Check sheet for the drawn part. Datum: minimum x, y, z corner. Units: mm. Give positions to 0.01 mm unless a question says otherwise; leave off trailing zeros. Order: outer loops, then holes, each group sorted by start corner. A loop starts at its lowest first (then second) coordinate and runs counter-clockwise, first axis right, second up. Notation, with made-up numbers: (37.25, -3.5) -> (82.25, -3.5) arc R10 cw to (82.25, 2.5) -> close; hole circle Ø2 at (57, 80.25). An arc over 180 degrees is marked (long way). Answer in a Markdown table with one row per item. Add a question column.
(1) Go/stop test with flat-tipped pins: pin 1 (5 mm diameter, centred on x = 25, z = 4.76, fed in from -Y); pin 2 (3.5 mm diameter, centred on x = 25, z = 29.3, fed in from +Y). Record where each tip stops, or that it passes through.
(2) Cross-section at B-B (z = 29.3). Record the cut outline in (x, y) (1 decimal), then the cut area to 3 significant figures.
(3) Thickness scan on L1, parallel to X at y = 5.5, z = 29; L2, parallel to Z at x = 42, y = 4.5 (1 decimal); L3, parallel to Z at x = 41.67, y = 6.5. Record the ranges inside material, lowest first. Write a range as [from, to].
(4) Cross-section at C-C (y = 7.75). State how many separate pieces and enclosed holes the cut face has, then the cut area to 3 significant figures.
(5) Cross-section at A-A (x = 41.67). Record the cut outline in (y, z) (1 decimal), then the cut area to 3 significant figures.
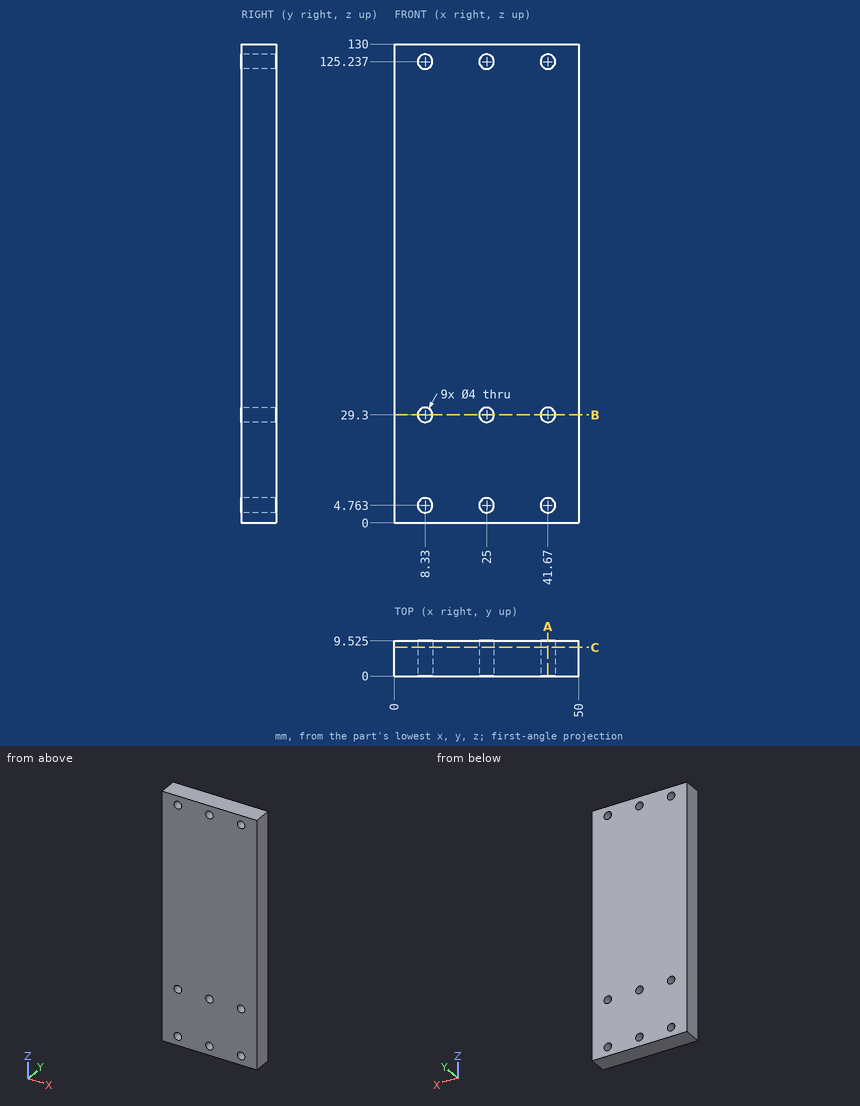
Answer below:
| question | item | result |
|---|---|---|
| 1 | pin 1 | stops at y = 0 |
| 1 | pin 2 | passes through |
| 2 | outline | (0, 0) -> (6.3, 0) -> (6.3, 9.5) -> (0, 9.5) -> close; (10.3, 0) -> (23, 0) -> (23, 9.5) -> (10.3, 9.5) -> close; (27, 0) -> (39.7, 0) -> (39.7, 9.5) -> (27, 9.5) -> close; (43.7, 0) -> (50, 0) -> (50, 9.5) -> (43.7, 9.5) -> close |
| 2 | area | 362 mm² |
| 3 | L1 | x = [0, 6.35], [10.31, 23.02], [26.98, 39.69], [43.65, 50] |
| 3 | L2 | z = [0, 2.8], [6.7, 27.3], [31.3, 123.3], [127.2, 130] |
| 3 | L3 | z = [0, 2.76], [6.76, 27.3], [31.3, 123.24], [127.24, 130] |
| 4 | separate pieces | 1 |
| 4 | enclosed holes | 9 |
| 4 | area | 6,390 mm² |
| 5 | outline | (0, 0) -> (9.5, 0) -> (9.5, 2.8) -> (0, 2.8) -> close; (0, 6.8) -> (9.5, 6.8) -> (9.5, 27.3) -> (0, 27.3) -> close; (0, 31.3) -> (9.5, 31.3) -> (9.5, 123.2) -> (0, 123.2) -> close; (0, 127.2) -> (9.5, 127.2) -> (9.5, 130) -> (0, 130) -> close |
| 5 | area | 1,120 mm² |
